Answer from the drawing. Dimensions are ordinates in mm from the lowest x, y and z of the part. Give positions to 0.01 mm unless a question says otherwise; leave off trailing zeros. Loops run counter-clockwise (first coordinate to the right, second up) from the corner with the lowest first, then second, coordinate; pieces in that order, holes last.
Item 1: Section C-C, the plane z = 178 is taken. Give the vertices of the cut face in (x, y) (1 decimal).
Item 2: Section B-B, the plane x = 1.25 is taken. Give the number of separate pieces and of enclosed holes in the cut face, and give its area (3 significant figures).
Item 3: Section A-A, the plane y = 101.6 is taken. Give the vertices of the cut face in (x, z).
Item 4: Section D-D, the plane y = 30 is taken. Give the vertices of the cut face in (x, z).
Item 5: Each of these flat-tipped pins is pushed along its axis until it touches: pin 1 Ø2 at (x, y) = (2.5, 106) entering from +Z; pin 2 Ø3.5 at (x, z) = (3, 110.5) entering from -Y; pin 3 Ø2 at (x, y) = (4.5, 98) entering from -Z. Where does it stop, or does it pass through?
Item 6: Consider line 1 along Z through (x, y) = (2.25, 82.55); line 2 along Z through (x, y) = (1, 119) (1 decimal); line 3 along Y through (x, z) = (3.5, 91.5). Determine where each line is inside the solid, lowest interval first.
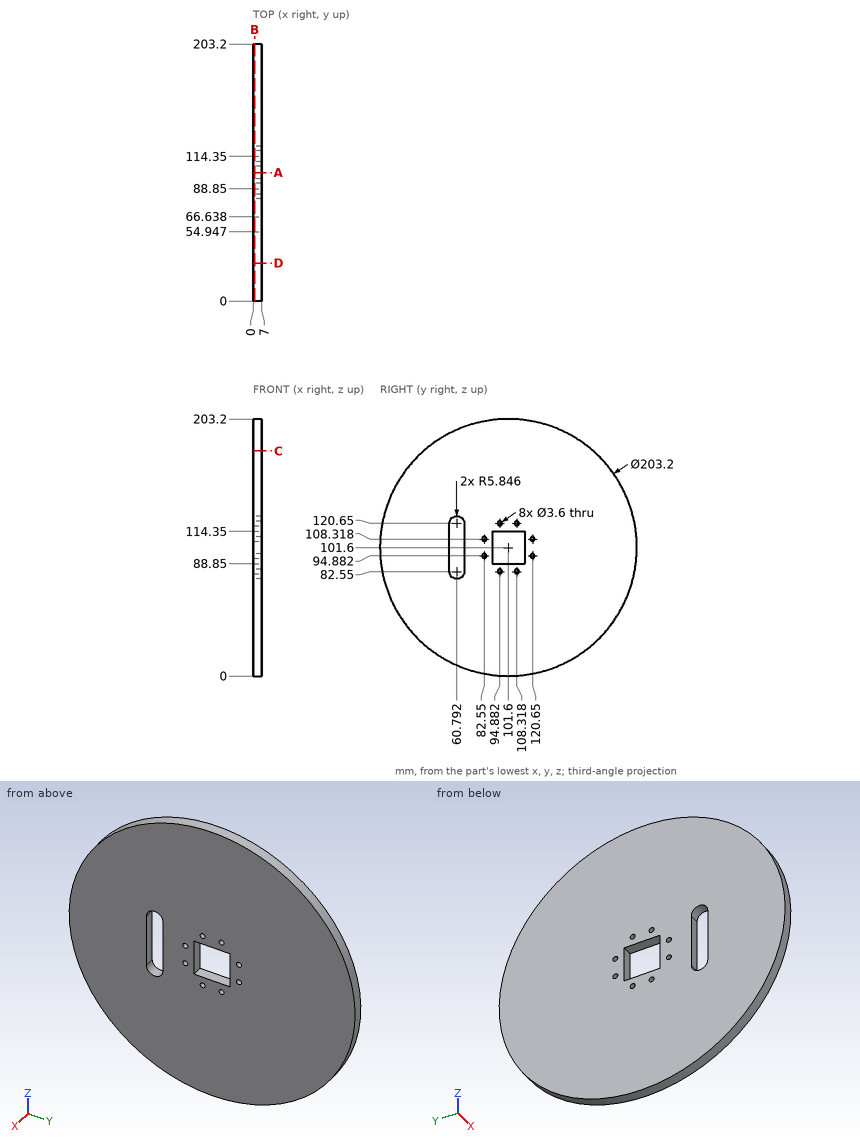
Worked answers:
1. outline: (0, 34.6) - (7, 34.6) - (7, 168.6) - (0, 168.6) - close
2. separate pieces: 1
2. enclosed holes: 10
2. area: 31,100 mm2
3. outline: (0, 0) - (7, 0) - (7, 88.85) - (0, 88.85) - close; (0, 114.35) - (7, 114.35) - (7, 203.2) - (0, 203.2) - close
4. outline: (0, 29.52) - (7, 29.52) - (7, 173.68) - (0, 173.68) - close
5. pin 1: stops at z = 203.14
5. pin 2: stops at y = 0.25
5. pin 3: stops at z = 0.03
6. line 1: z = 1.8 to 93.08, 96.68 to 106.52, 110.12 to 201.4
6. line 2: z = 1.5 to 94.2, 95.6 to 107.6, 109 to 201.7
6. line 3: y = 0.5 to 54.95, 66.64 to 88.85, 114.35 to 202.7
